Could you check a few things on this model? Use its own coordinates, in mm. A direction names the side the tool comes from. Round coordinates to 2 decimals unless told otherwise and drop trailing zeros. Loops run counter-clockwise (first coordinate to the right, second up) from the corner with the lowest first, then second, coordinate; pieces in that order, holes last. Notation, with made-up numbers: (0, 6.5) -> (16, 6.5) arc R24 ccw to (16, 43.5) -> close; hole circle Ø8 at (-10, -1.5). An arc over 180 degrees is marked (long way). One line per item, written item: value.
Solid Edge part; units mm, degrees
sketch "Sketch1" plane through (0, 0, 0) normal (0, -1, 0) x (1, 0, 0)
  line L0 (0, 40) -> (0, -40)
  arc A0 (0, 40) -> (0, -40) centre (0, 0) cw
revolve "RevolvedProtrusion1" add sketch "Sketch1" angle 360 about axis through (0, 0, 45) along (0, 0, -1)
sketch "Sketch2" plane through (0, 0, 0) normal (0, 0, 1) x (1, 0, 0)
  circle A0 centre (0, 0) radius 5.09
extrude "Protrusion1" add sketch "Sketch2" against normal blind 55
sketch "Sketch3" plane through (0, 0, -55) normal (0, 0, -1) x (1, 0, 0)
  line L0 (27.7128, 0) -> (13.8564, 24)
  line L1 (13.8564, 24) -> (-13.8564, 24)
  line L2 (-13.8564, 24) -> (-27.7128, 0)
  line L3 (-27.7128, 0) -> (-13.8564, -24)
  line L4 (-13.8564, -24) -> (13.8564, -24)
  line L5 (13.8564, -24) -> (27.7128, 0)
extrude "ExtrudedProtrusion_2" add sketch "Sketch3" along normal blind 4
(1) If we section it at D-D, the plane y = 32: Please give me the cut outline in (x, z).
Recorded:
outline: circle Ø48 at (0, 0)
(2) Thinking about a two-plate mould opening in Z: for faces 6 (the face through (0, 0, -59)), 7 (the face through (-6, 0, -55)), 8 (the face through (20.688, 12.168, -56.972)), which applies, released by +Z, released by -Z, zero draft, split by the parting line, or undercut?
Recorded:
face 6: released by -Z
face 7: undercut
face 8: zero draft
(3) If I drill on L1, parallel to Z at x = 16.5, y = -1.5; L2, parallel to Z at x = 10, y = 5.5; L3, parallel to Y at x = -26, z = 10.5, over which ranges is the centre line in solid material (lowest first)?
Recorded:
L1: -59 to -55, -36.41 to 36.41
L2: -59 to -55, -38.34 to 38.34
L3: -28.53 to 28.53
(4) If we section it at B-B, the plane x = -12.5: Please give me the cut outline in (y, z), then the cut area to 3 significant figures.
Recorded:
outline: circle Ø75.99 at (0, 0); (-24, -59) -> (24, -59) -> (24, -55) -> (-24, -55) -> close
area: 4,730 mm²
(5) If we section it at C-C, the plane z = -43.5: Please give me the cut outline in (x, y), then the cut area to 3 significant figures.
Recorded:
outline: circle Ø10.18 at (0, 0)
area: 81.4 mm²
(6) I'm going to push flat-ended pins straight in: pin 1 Ø4 at (x, z) = (25, -18) entering from -Y; pin 2 Ø6 at (x, z) = (-10, -15) entering from +Y; pin 3 Ø10 at (y, z) = (2, -22.5) entering from -X. Where does each tip first touch, or does it pass through?
Recorded:
pin 1: y = -27.75
pin 2: y = 37.07
pin 3: x = -35.93
(7) For faces 1 (the face through (20.9, -11.8, -57)), 2 (the face through (0, 24, -57)), 3 (the face through (-20.9, 11.8, -57)), 4 (the face through (-20.688, -12.168, -56.972)), 5 (the face through (0, -24, -57)), which set-ups out of +Z, -Z, +X, -X, +Y, -Y let a thin tool reach every point of the face, with its end or its side?
Recorded:
face 1: -Z, +X, -Y
face 2: -Z, +X, -X, +Y
face 3: -Z, -X, +Y
face 4: -Z, -X, -Y
face 5: -Z, +X, -X, -Y
(8) If we section it at A-A, the plane x = 0: Please give me the cut outline in (y, z), then the cut area to 3 significant figures.
Recorded:
outline: (-24, -59) -> (24, -59) -> (24, -55) -> (5.09, -55) -> (5.09, -39.67) arc R40 ccw (long way) to (-5.09, -39.67) -> (-5.09, -55) -> (-24, -55) -> close
area: 5,370 mm²
